```python
from build123d import *

# Parameters (mm, degrees)
F1_DEPTH = 44
F2_W     = 120
F2_H     = 120
F3_DEPTH = 22
F4_W     = 120
F4_H     = 120
F5_DEPTH = 22


with BuildPart() as f1:
    # F0 (on Top) → F1 (new body)
    with BuildSketch(Plane.XY):
        with BuildLine():
            Line((-120, 0), (0, 0))
            Line((0, 0), (0, 650))
            ThreePointArc((0, 650), (-58.578644, 791.421356), (-200, 850))
            Line((-200, 850), (-350, 850))
            Line((-350, 850), (-350, 730))
            Line((-350, 730), (-200, 730))
            ThreePointArc((-200, 730), (-143.431458, 706.568542), (-120, 650))
            Line((-120, 650), (-120, 0))
        make_face()
    extrude(amount=F1_DEPTH)

    # F2 (on face) → F3 (cut)
    with BuildSketch(Plane(origin=(0, 0, 0), x_dir=(1, 0, 0), z_dir=(0, 0, -1))):
        with Locations((-60, -60)):
            Rectangle(F2_W, F2_H)
    extrude(amount=-F3_DEPTH, mode=Mode.SUBTRACT)

    # F4 (on face) → F5 (cut)
    with BuildSketch(Plane(origin=(0, 0, 0), x_dir=(1, 0, 0), z_dir=(0, 0, -1))):
        with Locations((-290, -790)):
            Rectangle(F4_W, F4_H)
    extrude(amount=-F5_DEPTH, mode=Mode.SUBTRACT)


solid = f1.part
```
Check sheet for the modelled part. Datum: model origin and axes. Units: mm. A direction names the side the tool comes from. Round coordinates to 2 decimals unless told otherwise and drop trailing zeros. Loops run counter-clockwise (first coordinate to the right, second up) from the corner with the lowest first, then second, coordinate; pieces in that order, holes last. Notation, with made-up numbers: (-5, -22) - (11, -22) arc R21 cw to (11, 11) - close; hole circle Ø1 at (65, 43.5). An arc over 180 degrees is marked (long way). Answer as a JSON object with one key per item and string values. Group by question number.
Q1. Sectioned sample at C-C, the plane y = 799. Enter the section's corners in (x, z).
Q2. Sectioned sample at D-D, the plane x = -25. Enter the section's corners in (y, z), plus the area to 3 significant figures.
Q3. Scan lines: line 1 along X through (y, z) = (390.5, 23.5); line 2 along Y through (x, z) = (-239.5, 27); line 3 along Y through (x, z) = (-176, 6). Record each from-to range of solid material in increasing order. Write a range as [from, to].
Q4. Sectioned sample at B-B, the plane x = -271. Enter the section's corners in (y, z), plus the area to 3 significant figures.
Q5. Set-up check for faces 1 (the face through (-230, 791, 11)), 2 (the face through (-61, 120, 11)), 3 (the face through (-259, 730, 31)): record each of +Z, -Z, +X, -X, +Y, -Y from which the full face is reachable in a straight line by a thin tool's end or side.
Q6. Gauge pin test, flat ends, axial feed: P1, Ø10, axis at y = 371, z = 13, coming from the +X side; P2, Ø6, axis at y = 707.5, z = 13, coming from the +X side; P3, Ø13, axis at y = 239.5, z = 31, coming from the -X side; P4, Ø17.5, axis at y = 772.5, z = 9.5, coming from the -X side. Record the tip position at first contact, or that the pin passes through.
Q7. Sectioned sample at A-A, the plane z = 32. Enter the section's corners in (x, y), plus the area to 3 significant figures.
Solution:
{
 "1": {"outline": "(-350, 22) - (-230, 22) - (-230, 0) - (-66.59, 0) - (-66.59, 44) - (-350, 44) - close"},
 "2": {"outline": "(0, 22) - (120, 22) - (120, 0) - (746.82, 0) - (746.82, 44) - (0, 44) - close", "area": "30,200 mm²"},
 "3": {"line 1": "x = [-120, 0]", "line 2": "y = [730, 850]", "line 3": "y = [726.32, 848.55]"},
 "4": {"outline": "(730, 22) - (850, 22) - (850, 44) - (730, 44) - close", "area": "2,640 mm²"},
 "5": {"face 1": "-Z, -X, +Y, -Y", "face 2": "-Z, +X, -X, -Y", "face 3": "+Z, -Z, -X, -Y"},
 "6": {"P1": "stops at x = 0", "P2": "stops at x = -7.57", "P3": "stops at x = -120", "P4": "stops at x = -230"},
 "7": {"outline": "(-350, 730) - (-200, 730) arc R80 cw to (-120, 650) - (-120, 0) - (0, 0) - (0, 650) arc R200 ccw to (-200, 850) - (-350, 850) - close", "area": "122,000 mm²"}
}
